Answer from the drawing. Dimensions are ordinates in mm from the lowest x, y and z of the part. A direction names the side the tool comes from. Give positions to 0.01 mm unless a question says otherwise; leave off trailing zeros. Write each loop counter-clockwise with the first axis right and the second up, starting at its lowest first coordinate (ties: lowest second). Pieces come first, ordered by that corner, then holes. Notation, with made-up numbers: (3, -12) - (62, -12) arc R29 cw to (62, 18) - close; hole circle Ø8 at (39.5, -24.75). An arc over 180 degrees is marked (long way). Answer as a JSON object with one key per item and string values. Group by question number.
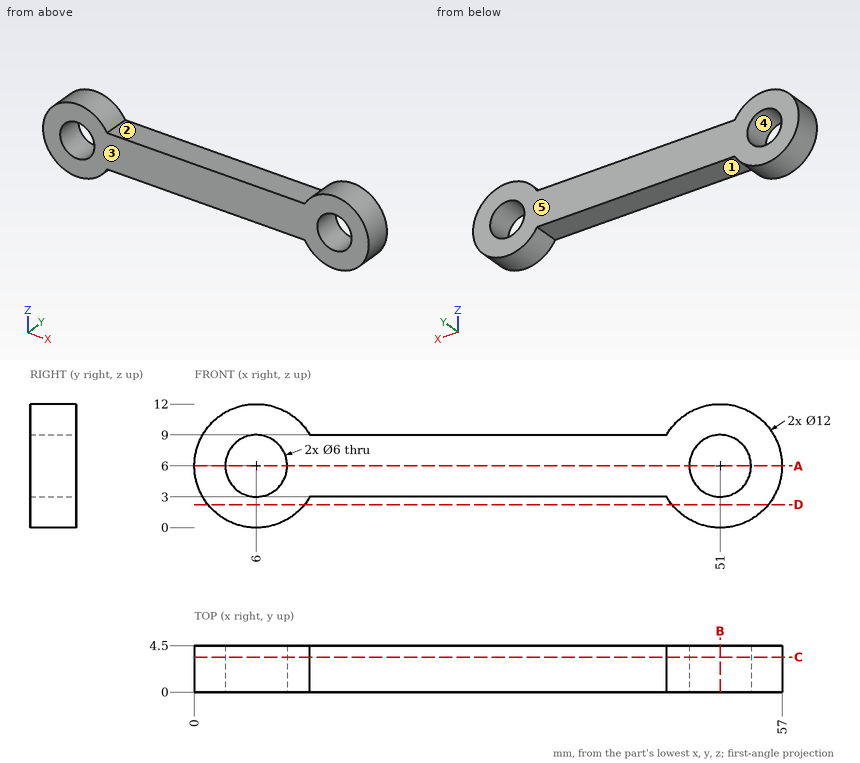
1) For a pull along X with two mould halves and no side action, classify the marked faces 4 and 5 as released by +X, released by -X, zero draft, split by the parting line, or undercut.
2) Find the intervals of material crossed by line 1 (X direction, y = 1.75, z = 6.25); line 2 (Z direction, x = 51, y = 2.1); line 3 (X direction, y = 4.2, z = 8.75), in increasing order. Write a range as [from, to].
3) Find section D-D, the plane z = 2.25. Write down the section's boundary in (x, y).
4) Which of the six approach directions +Z, -Z, +X, -X, +Y, -Y give full straight-line access (tool end or side, diameter ignored) to the marked faces 1, 2 and 3?
5) Flat-ended cylindrical pins translate along their axes: pin 1 Ø1 at (y, z) = (3, 8.5) entering from -X; pin 2 Ø1.3 at (x, y) = (23, 1.5) entering from -Z; pin 3 Ø2 at (y, z) = (2.5, 10.5) entering from -X. Find the tip coordinate at first contact, or state that the pin passes through.
6) Find section A-A, the plane z = 6. Write down the section's boundary in (x, y).
7) Find section C-C, the plane y = 3.4. Write down the section's boundary in (x, z).
8) Find section B-B, the plane x = 51. Write down the section's boundary in (y, z).
Values follow:
{
 "1": {"face 4": "undercut", "face 5": "zero draft"},
 "2": {"line 1": "x = [0.01, 3.01], [8.99, 48.01], [53.99, 56.99]", "line 2": "z = [0, 3], [9, 12]", "line 3": "x = [0.67, 4.8], [7.2, 49.8], [52.2, 56.33]"},
 "3": {"outline": "(1.32, 0) - (10.68, 0) - (10.68, 4.5) - (1.32, 4.5) - close; (46.32, 0) - (55.68, 0) - (55.68, 4.5) - (46.32, 4.5) - close"},
 "4": {"face 1": "-Z, +Y, -Y", "face 2": "+Z, +Y, -Y", "face 3": "+Z, -Z, +X, -X, -Y"},
 "5": {"pin 1": "stops at x = 0.34", "pin 2": "stops at z = 3", "pin 3": "stops at x = 1.13"},
 "6": {"outline": "(0, 0) - (3, 0) - (3, 4.5) - (0, 4.5) - close; (9, 0) - (48, 0) - (48, 4.5) - (9, 4.5) - close; (54, 0) - (57, 0) - (57, 4.5) - (54, 4.5) - close"},
 "7": {"outline": "(11.2, 3) - (45.8, 3) arc R6 ccw (long way) to (45.8, 9) - (11.2, 9) arc R6 ccw (long way) to start; hole circle Ø6 at (6, 6); hole circle Ø6 at (51, 6)"},
 "8": {"outline": "(0, 0) - (4.5, 0) - (4.5, 3) - (0, 3) - close; (0, 9) - (4.5, 9) - (4.5, 12) - (0, 12) - close"}
}
